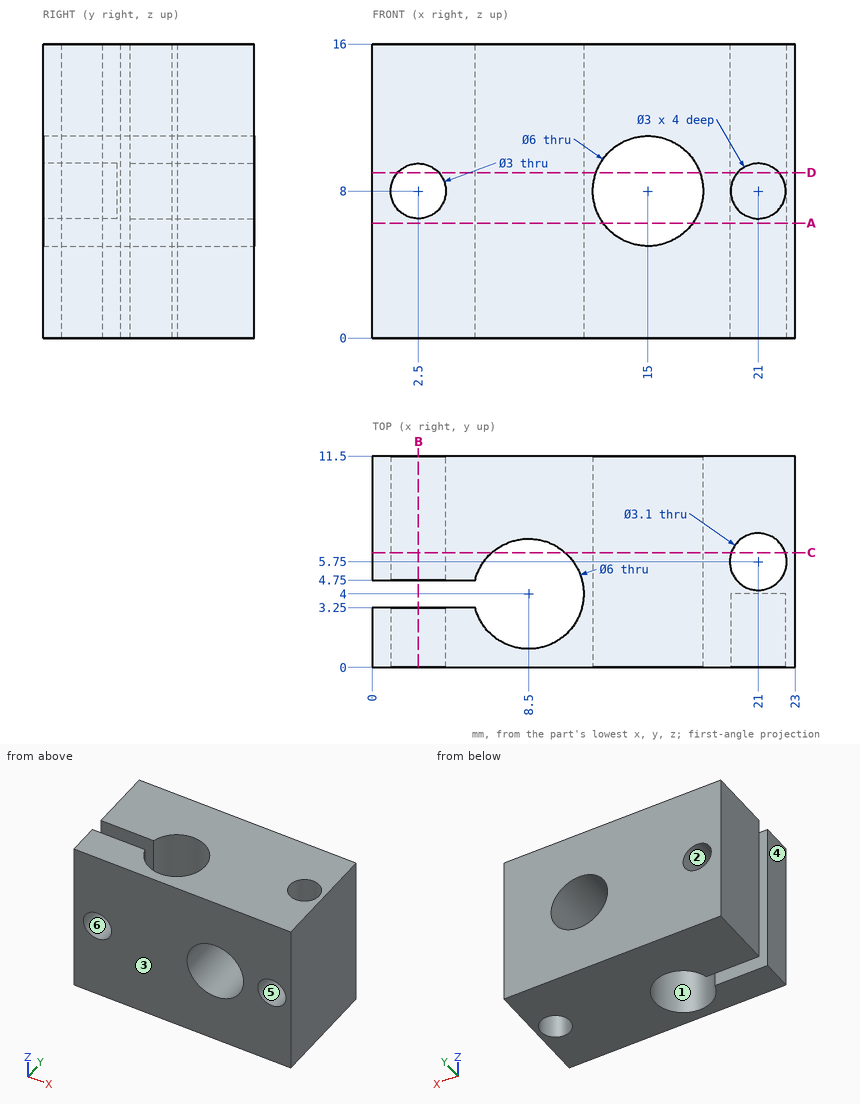
Verification items for this drawing (mm, ordinates from the low corner). A direction names the side the tool comes from. Give positions to 0.01 mm unless a question says otherwise; leave off trailing zeros. Loops run counter-clockwise (first coordinate to the right, second up) from the corner with the lowest first, then second, coordinate; pieces in that order, holes last.
1. Tool access check on the marked faces 5 and 6. Record the directions out of +Z, -Z, +X, -X, +Y, -Y that give a thin tool (end or side, any length) a straight path to the whole face; none if there is none.
Derived:
face 5: -Y
face 6: +Y, -Y
2. Cross-section at C-C on y = 6.25. Record the cut outline in (x, z), and give its area (3 significant figures).
Derived:
outline: (0, 0) - (6.52, 0) - (6.52, 16) - (0, 16) - close; (10.48, 0) - (19.53, 0) - (19.53, 16) - (10.48, 16) - close; (22.47, 0) - (23, 0) - (23, 16) - (22.47, 16) - close; hole circle Ø3 at (2.5, 8); hole circle Ø6 at (15, 8)
area: 222 mm2
3. Cross-section at D-D on z = 9. Record the cut outline in (x, y), and give its area (3 significant figures).
Derived:
outline: (0, 0) - (1.38, 0) - (1.38, 3.25) - (0, 3.25) - close; (0, 4.75) - (1.38, 4.75) - (1.38, 11.5) - (0, 11.5) - close; (3.62, 0) - (12.17, 0) - (12.17, 11.5) - (3.62, 11.5) - (3.62, 4.75) - (5.6, 4.75) arc R3 cw (long way) to (5.6, 3.25) - (3.62, 3.25) - close; (17.83, 0) - (19.88, 0) - (19.88, 4) - (22.12, 4) - (22.12, 0) - (23, 0) - (23, 11.5) - (17.83, 11.5) - close; hole circle Ø3.1 at (21, 5.75)
area: 124 mm2
4. Cross-section at A-A on z = 6.25. Record the cut outline in (x, y), and give its area (3 significant figures).
Derived:
outline: (0, 0) - (12.56, 0) - (12.56, 11.5) - (0, 11.5) - (0, 4.75) - (5.6, 4.75) arc R3 cw (long way) to (5.6, 3.25) - (0, 3.25) - close; (17.44, 0) - (23, 0) - (23, 11.5) - (17.44, 11.5) - close; hole circle Ø3.1 at (21, 5.75)
area: 164 mm2
5. Cross-section at B-B on x = 2.5. Record the cut outline in (y, z), and give its area (3 significant figures).
Derived:
outline: (0, 0) - (3.25, 0) - (3.25, 6.5) - (0, 6.5) - close; (0, 9.5) - (3.25, 9.5) - (3.25, 16) - (0, 16) - close; (4.75, 0) - (11.5, 0) - (11.5, 6.5) - (4.75, 6.5) - close; (4.75, 9.5) - (11.5, 9.5) - (11.5, 16) - (4.75, 16) - close
area: 130 mm2
6. Release check for a two-part mould opening along X. For the marked faces 1, 2, 3 and 4 record: +X half, -X half, draft (parallel to the pull), parting line (faces both ways), or undercut.
Derived:
face 1: undercut
face 2: undercut
face 3: draft
face 4: -X half
7. Material ranges on probe 1 along Y at (x, z) = (3.25, 5); probe 2 along X at (y, z) = (5.25, 12.75); probe 3 along X at (y, z) = (5.25, 8.25), recorded low to high.
Derived:
probe 1: y = 0 to 3.25, 4.75 to 11.5
probe 2: x = 0 to 5.77, 11.23 to 19.53, 22.47 to 23
probe 3: x = 0 to 1.02, 3.98 to 5.77, 11.23 to 12.01, 17.99 to 19.53, 22.47 to 23
